For this review, take the finished solid that the model builds, in its own axes (mm). Face numbers are marked on the shaded views. A direction names the side the tool comes from. Coordinates: 2 decimals unless noted, no trailing zeros. Order: outer loops, then holes, each group sorted by start corner. A loop starts at its lowest first (then second) coordinate and runs counter-clockwise, first axis right, second up. Notation, with made-up numbers: (62, -26) -> (75, -26) arc R30 ccw to (75, 2) -> close; hole circle Ø7 at (-20.75, 70.5). An arc over 180 degrees is marked (long way). Return JSON: item names as keys, results as strings. Group by question number.
Item 1: Draft analysis for pull direction X (two halves, no side actions). For the marked faces 4, 5, 6 and 7, state which applies: +X half, -X half, draft (parallel to the pull), parting line (faces both ways), or undercut.
Item 2: Machinability: for the marked faces 1, 2 and 3, which of the approach directions +Z, -Z, +X, -X, +Y, -Y give a long, thin tool a straight path to every point of the face, cutting with its end or side? Answer none if there is none.
Item 3: Insertion check: pin 1 (6.5 mm diameter, centred on x = 14, z = 4, fed in from -Y); pin 2 (5 mm diameter, centred on y = -19, z = 0, fed in from +X); pin 3 (2.5 mm diameter, centred on x = -11.5, z = 5, fed in from +Y). Each pin has a flat end and moves straight along its axis. Give the tip position at first contact, or say it passes through.
Item 4: Take a section at A-A (y = 0). Write out the cut boundary in (x, z).
Item 5: For line 1 along Y through (x, z) = (0, 4.5); line 2 along X through (y, z) = (34.5, 4.5); line 3 along Y through (x, z) = (-6.5, 0.5), list the stretches that pass through material, from the lowest coordinate up.
Item 6: Take a section at C-C (z = -4). Write out the cut boundary in (x, y), then the cut area to 3 significant figures.
Item 7: Take a section at D-D (y = -31). Write out the cut boundary in (x, z).
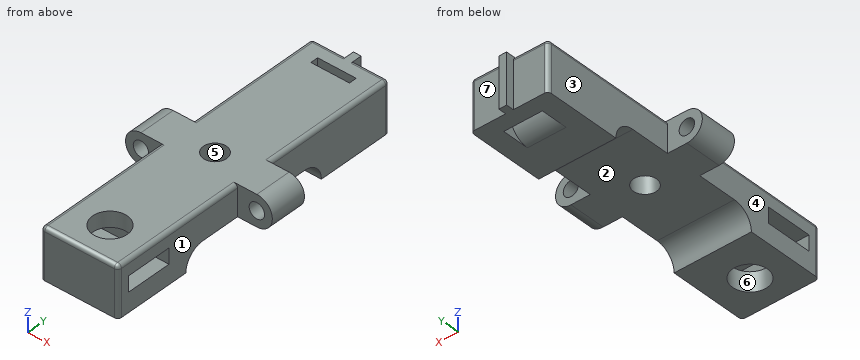
```python
from build123d import *

# Parameters (mm, degrees)
BOSS_EXTRUDE1_DEPTH      = 10
SKETCH7_R                = 2
BOSS_EXTRUDE4_DEPTH      = 4.75
SKETCH8_R                = 3
CUT_EXTRUDE1_DEPTH       = 8
FILLET1_R                = 1
M8_CLEARANCE_HOLE1_D     = 9
FILLET2_R                = 5
SKETCH15_W               = 4
SKETCH15_H               = 12
CUT_EXTRUDE2_DEPTH       = 20
SKETCH16_W               = 10
SKETCH16_H               = 2
CUT_EXTRUDE3_DEPTH       = 47.151923037
FILLET3_R                = 5
BOSS_EXTRUDE5_DEPTH      = 2
BOSS_EXTRUDE5_DEPTH_BACK = 2
SKETCH17_W               = 2
SKETCH17_H               = 13


with BuildPart() as part:
    # Sketch1 → Boss-Extrude1 (new, symmetric)
    with BuildSketch(Plane(origin=(0, 0, 0), x_dir=(0, 0, -1), z_dir=(1, 0, 0))):
        Polygon((0, -20), (0, 20), (5, 20), (5, 40), (-8, 40), (-8, 20), (-8, -20), (-8, -40), (5, -40), (5, -20), align=None)
    extrude(amount=BOSS_EXTRUDE1_DEPTH, both=True)

    # Sketch7 → Boss-Extrude4 (add, symmetric)
    # profile 1 of 2: a face of its own
    with BuildSketch(Plane(origin=(0, 0, 0), x_dir=(1, 0, 0), z_dir=(0, 1, 0))):
        with BuildLine():
            Line((-15, 0), (-10, 0))
            Line((-10, 0), (-10, -8))
            Line((-10, -8), (-15, -8))
            ThreePointArc((-15, -8), (-19, -4), (-15, 0))
        make_face()
        with Locations(Location((-15, -4, 0), (0, 0, 270))):
            Circle(SKETCH7_R, mode=Mode.SUBTRACT)
    # profile 2 of 2: a face of its own
    with BuildSketch(Plane(origin=(0, 0, 0), x_dir=(1, 0, 0), z_dir=(0, 1, 0))):
        with BuildLine():
            Line((15, -8), (10, -8))
            Line((10, -8), (10, 0))
            Line((10, 0), (15, 0))
            ThreePointArc((15, 0), (19, -4), (15, -8))
        make_face()
        with Locations(Location((15, -4, 0), (0, 0, 90))):
            Circle(SKETCH7_R, mode=Mode.SUBTRACT)
    extrude(amount=BOSS_EXTRUDE4_DEPTH, both=True)

    # Sketch8 → Cut-Extrude1 (cut)
    with BuildSketch(Plane(origin=(0, 0, 0), x_dir=(-1, 0, 0), z_dir=(0, 0, -1))):
        Circle(SKETCH8_R)
    extrude(amount=-CUT_EXTRUDE1_DEPTH, mode=Mode.SUBTRACT)

    # Fillet1
    fillet1_edges = [part.edges().sort_by_distance(p)[0] for p in [
        (-10, -40, 1.5),
        (10, -40, 1.5),
        (-10, 40, 1.5),
        (10, 40, 1.5),
        (0, -40, 8),
        (-10, -22.375, 8),
        (10, -22.375, 8),
        (10, 22.375, 8),
        (0, 40, 8),
        (-10, 22.375, 8),
    ]]
    fillet(fillet1_edges, radius=FILLET1_R)

    # M8 Clearance Hole1 (through all)
    with Locations(Plane(origin=(0, -31, -5), x_dir=(-1, 0, 0), z_dir=(0, 0, -1))):
        with Locations((0, 0)):
            Hole(M8_CLEARANCE_HOLE1_D / 2)

    # Fillet2
    fillet2_edges = [part.edges().sort_by_distance(p)[0] for p in [
        (0, 20, 0),
        (0, -20, 0),
    ]]
    fillet(fillet2_edges, radius=FILLET2_R - 0.0001)  # a hair under: the kernel refuses the full size

    # Sketch15 → Cut-Extrude2 (cut)
    with BuildSketch(Plane.ZY.offset(10)):
        with Locations((2, -31)):
            Rectangle(SKETCH15_W, SKETCH15_H)
    extrude(amount=-CUT_EXTRUDE2_DEPTH, mode=Mode.SUBTRACT)

    # Sketch16 → Cut-Extrude3 (cut, through all)
    with BuildSketch(Plane.XY.offset(8)):
        with Locations((0, 35)):
            Rectangle(SKETCH16_W, SKETCH16_H)
    extrude(amount=-CUT_EXTRUDE3_DEPTH, mode=Mode.SUBTRACT)

    # Fillet3
    fillet3_edges = [part.edges().sort_by_distance(p)[0] for p in [
        (0, 34, -5),
    ]]
    fillet(fillet3_edges, radius=FILLET3_R)

    # Sketch17 → Boss-Extrude5 (add, two sides: drawn at the far end of the back side and taken through both)
    with BuildSketch(Plane(origin=(0, 40, 0), x_dir=(1, 0, 0), z_dir=(0, 1, 0)).offset(-BOSS_EXTRUDE5_DEPTH_BACK)):
        with Locations((0, -1.5)):
            Rectangle(SKETCH17_W, SKETCH17_H)
    extrude(amount=BOSS_EXTRUDE5_DEPTH + BOSS_EXTRUDE5_DEPTH_BACK)


solid = part.part
```
Findings below:
{
 "1": {"face 4": "-X half", "face 5": "undercut", "face 6": "undercut", "face 7": "draft"},
 "2": {"face 1": "+Z, -Z, +X, -Y", "face 2": "-Z, +X, -X", "face 3": "+Z, -Z, -X, +Y"},
 "3": {"pin 1": "stops at y = -4.75", "pin 2": "stops at x = 10", "pin 3": "stops at y = 4.75"},
 "4": {"outline": "(-15, 0) -> (-3, 0) -> (-3, 8) -> (-15, 8) arc R4 ccw to start; (3, 0) -> (15, 0) arc R4 ccw to (15, 8) -> (3, 8) -> close; hole circle Ø4 at (-15, 4); hole circle Ø4 at (15, 4)"},
 "5": {"line 1": "y = -40 to -35.5, -26.5 to -3, 3 to 34, 36 to 42", "line 2": "x = -10 to -5, 5 to 10", "line 3": "y = -40 to -37, -25 to 40"},
 "6": {"outline": "(-10, -39) arc R1 ccw to (-9, -40) -> (9, -40) arc R1 ccw to (10, -39) -> (10, -19.9) -> (-10, -19.9) -> close; (-10, 19.9) -> (10, 19.9) -> (10, 39) arc R1 ccw to (9, 40) -> (1, 40) -> (1, 42) -> (-1, 42) -> (-1, 40) -> (-9, 40) arc R1 ccw to (-10, 39) -> close; hole (-5, 32) -> (5, 32) -> (5, 36) -> (-5, 36) -> close; hole circle Ø9 at (0, -31)", "area": "704 mm2"},
 "7": {"outline": "(-10, -5) -> (-4.5, -5) -> (-4.5, 0) -> (-10, 0) -> close; (-10, 4) -> (-4.5, 4) -> (-4.5, 8) -> (-9, 8) arc R1 ccw to (-10, 7) -> close; (4.5, -5) -> (10, -5) -> (10, 0) -> (4.5, 0) -> close; (4.5, 4) -> (10, 4) -> (10, 7) arc R1 ccw to (9, 8) -> (4.5, 8) -> close"}
}
